Here's how the part is built. I have some questions about the finished solid (model axes, mm). Coordinates: 2 decimals unless noted, no trailing zeros. Loops run counter-clockwise (first coordinate to the right, second up) from the corner with the lowest first, then second, coordinate; pieces in that order, holes last. Notation, with made-up numbers: (52.5, -19) -> (109.5, -19) arc R6 ccw to (109.5, -12) -> close; hole circle Ø3 at (-16.75, -18). An arc over 180 degrees is marked (long way). Answer as a JSON object with one key per item and string values. Group by question number.
1) I want a section at B-B (x = 70). Write out the boundary of the cut face in (y, z), then the cut area to 3 significant figures.
2) I want a section at A-A (z = -120.5). Write out the boundary of the cut face in (x, y), then the cut area to 3 significant figures.
3) I want a section at C-C (y = -0.95). Count the separate pieces of the cut face and the enclosed holes in it, then the cut area to 3 significant figures.
4) I need wall thicknesses on probe 1 along X at (y, z) = (-0.5, -60); probe 2 along X at (y, z) = (-1.2, -145); probe 3 along Z at (x, y) = (181, -1.1). Which ranges of each line are inside material? Lowest first, please. Write a range as [from, to].
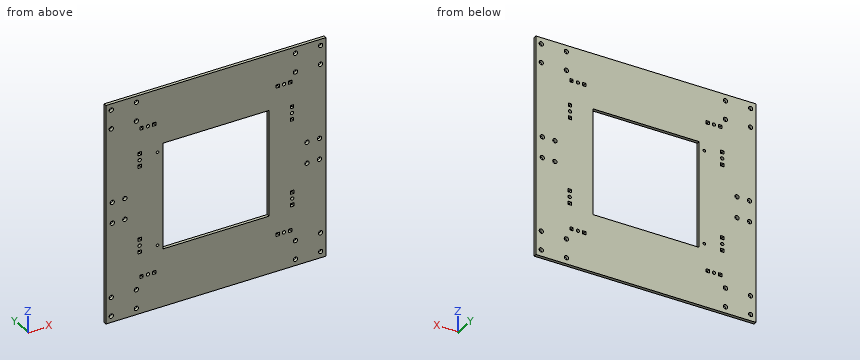
```python
from build123d import *

# Parameters (mm, degrees)
SKETCH2_W           = 210
SKETCH2_H           = 210
SKETCH2_R           = 2.05
SKETCH2_R_2         = 1.575
SKETCH2_R_3         = 1.25
SKETCH2_W_2         = 101.6
SKETCH2_H_2         = 101.6
SKETCH2_W_3         = 3.15
SKETCH2_H_3         = 3.15
BOSS_EXTRUDE2_DEPTH = 3


with BuildPart() as part:
    # Sketch2 → Boss-Extrude2 (new body)
    with BuildSketch(Plane(origin=(0, 0, 0), x_dir=(1, 0, 0), z_dir=(0, 1, 0))):
        with Locations((105, 105)):
            Rectangle(SKETCH2_W, SKETCH2_H)
        with Locations(Location((5, 24, 0), (0, 0, 270))):
            Circle(SKETCH2_R, mode=Mode.SUBTRACT)
        with Locations(Location((29, 24, 0), (0, 0, 270))):
            Circle(SKETCH2_R, mode=Mode.SUBTRACT)
        with Locations(Location((40, 32.3, 0), (0, 0, 270))):
            Circle(SKETCH2_R_2, mode=Mode.SUBTRACT)
        with Locations(Location((205, 6, 0), (0, 0, 270))):
            Circle(SKETCH2_R, mode=Mode.SUBTRACT)
        with Locations(Location((181, 6, 0), (0, 0, 270))):
            Circle(SKETCH2_R, mode=Mode.SUBTRACT)
        with Locations(Location((170, 32.3, 0), (0, 0, 270))):
            Circle(SKETCH2_R_2, mode=Mode.SUBTRACT)
        with Locations(Location((29, 6, 0), (0, 0, 270))):
            Circle(SKETCH2_R, mode=Mode.SUBTRACT)
        with Locations(Location((5, 6, 0), (0, 0, 270))):
            Circle(SKETCH2_R, mode=Mode.SUBTRACT)
        with Locations(Location((181, 24, 0), (0, 0, 270))):
            Circle(SKETCH2_R, mode=Mode.SUBTRACT)
        with Locations(Location((205, 24, 0), (0, 0, 270))):
            Circle(SKETCH2_R, mode=Mode.SUBTRACT)
        with Locations(Location((205, 186, 0), (0, 0, 270))):
            Circle(SKETCH2_R, mode=Mode.SUBTRACT)
        with Locations(Location((181, 186, 0), (0, 0, 270))):
            Circle(SKETCH2_R, mode=Mode.SUBTRACT)
        with Locations(Location((40, 174.76, 0), (0, 0, 270))):
            Circle(SKETCH2_R_2, mode=Mode.SUBTRACT)
        with Locations(Location((181, 204, 0), (0, 0, 270))):
            Circle(SKETCH2_R, mode=Mode.SUBTRACT)
        with Locations(Location((205, 204, 0), (0, 0, 270))):
            Circle(SKETCH2_R, mode=Mode.SUBTRACT)
        with Locations(Location((5, 204, 0), (0, 0, 270))):
            Circle(SKETCH2_R, mode=Mode.SUBTRACT)
        with Locations(Location((29, 204, 0), (0, 0, 270))):
            Circle(SKETCH2_R, mode=Mode.SUBTRACT)
        with Locations(Location((170, 174.76, 0), (0, 0, 270))):
            Circle(SKETCH2_R_2, mode=Mode.SUBTRACT)
        with Locations(Location((29, 186, 0), (0, 0, 270))):
            Circle(SKETCH2_R, mode=Mode.SUBTRACT)
        with Locations(Location((5, 186, 0), (0, 0, 270))):
            Circle(SKETCH2_R, mode=Mode.SUBTRACT)
        with Locations(Location((177.6, 62.41, 0), (0, 0, 270))):
            Circle(SKETCH2_R_2, mode=Mode.SUBTRACT)
        with Locations(Location((177.88, 144.65, 0), (0, 0, 270))):
            Circle(SKETCH2_R_2, mode=Mode.SUBTRACT)
        with Locations(Location((32.12, 144.65, 0), (0, 0, 270))):
            Circle(SKETCH2_R_2, mode=Mode.SUBTRACT)
        with Locations(Location((32.12, 62.41, 0), (0, 0, 270))):
            Circle(SKETCH2_R_2, mode=Mode.SUBTRACT)
        with Locations(Location((49.2, 149.719, 0), (0, 0, 270))):
            Circle(SKETCH2_R_3, mode=Mode.SUBTRACT)
        with Locations(Location((49.2, 60.281, 0), (0, 0, 270))):
            Circle(SKETCH2_R_3, mode=Mode.SUBTRACT)
        with Locations(Location((18.000065795, 95, 0), (0, 0, 270))):
            Circle(SKETCH2_R, mode=Mode.SUBTRACT)
        with Locations(Location((18, 115, 0), (0, 0, 270))):
            Circle(SKETCH2_R, mode=Mode.SUBTRACT)
        with Locations(Location((6, 115.000053284, 0), (0, 0, 270))):
            Circle(SKETCH2_R, mode=Mode.SUBTRACT)
        with Locations(Location((6, 95, 0), (0, 0, 270))):
            Circle(SKETCH2_R, mode=Mode.SUBTRACT)
        with Locations(Location((204, 95, 0), (0, 0, 270))):
            Circle(SKETCH2_R, mode=Mode.SUBTRACT)
        with Locations(Location((204, 115.000053284, 0), (0, 0, 270))):
            Circle(SKETCH2_R, mode=Mode.SUBTRACT)
        with Locations(Location((191.999934205, 95, 0), (0, 0, 270))):
            Circle(SKETCH2_R, mode=Mode.SUBTRACT)
        with Locations(Location((192, 115, 0), (0, 0, 270))):
            Circle(SKETCH2_R, mode=Mode.SUBTRACT)
        with Locations((105, 103.919)):
            Rectangle(SKETCH2_W_2, SKETCH2_H_2, mode=Mode.SUBTRACT)
        with Locations((32.12, 150.725)):
            Rectangle(SKETCH2_W_3, SKETCH2_H_3, mode=Mode.SUBTRACT)
        with Locations((32.12, 138.575)):
            Rectangle(SKETCH2_W_3, SKETCH2_H_3, mode=Mode.SUBTRACT)
        with Locations((32.12, 68.485)):
            Rectangle(SKETCH2_W_3, SKETCH2_H_3, mode=Mode.SUBTRACT)
        with Locations((32.12, 56.335)):
            Rectangle(SKETCH2_W_3, SKETCH2_H_3, mode=Mode.SUBTRACT)
        with Locations((177.6, 68.485)):
            Rectangle(SKETCH2_W_3, SKETCH2_H_3, mode=Mode.SUBTRACT)
        with Locations((177.6, 56.335)):
            Rectangle(SKETCH2_W_3, SKETCH2_H_3, mode=Mode.SUBTRACT)
        with Locations((177.88, 138.575)):
            Rectangle(SKETCH2_W_3, SKETCH2_H_3, mode=Mode.SUBTRACT)
        with Locations((177.88, 150.725)):
            Rectangle(SKETCH2_W_3, SKETCH2_H_3, mode=Mode.SUBTRACT)
        with Locations((33.925, 32.3)):
            Rectangle(SKETCH2_W_3, SKETCH2_H_3, mode=Mode.SUBTRACT)
        with Locations((46.075, 32.3)):
            Rectangle(SKETCH2_W_3, SKETCH2_H_3, mode=Mode.SUBTRACT)
        with Locations((33.925, 174.76)):
            Rectangle(SKETCH2_W_3, SKETCH2_H_3, mode=Mode.SUBTRACT)
        with Locations((46.075, 174.76)):
            Rectangle(SKETCH2_W_3, SKETCH2_H_3, mode=Mode.SUBTRACT)
        with Locations((176.075, 32.3)):
            Rectangle(SKETCH2_W_3, SKETCH2_H_3, mode=Mode.SUBTRACT)
        with Locations((163.925, 32.3)):
            Rectangle(SKETCH2_W_3, SKETCH2_H_3, mode=Mode.SUBTRACT)
        with Locations((163.925, 174.76)):
            Rectangle(SKETCH2_W_3, SKETCH2_H_3, mode=Mode.SUBTRACT)
        with Locations((176.075, 174.76)):
            Rectangle(SKETCH2_W_3, SKETCH2_H_3, mode=Mode.SUBTRACT)
    extrude(amount=-BOSS_EXTRUDE2_DEPTH)


solid = part.part
```
Determined:
{
 "1": {"outline": "(-3, -210) -> (0, -210) -> (0, -154.72) -> (-3, -154.72) -> close; (-3, -53.12) -> (0, -53.12) -> (0, 0) -> (-3, 0) -> close", "area": "325 mm^2"},
 "2": {"outline": "(0, -3) -> (54.2, -3) -> (54.2, 0) -> (0, 0) -> close; (155.8, -3) -> (210, -3) -> (210, 0) -> (155.8, 0) -> close", "area": "325 mm^2"},
 "3": {"separate pieces": "1", "enclosed holes": "51", "area": "33,200 mm^2"},
 "4": {"probe 1": "[0, 47.98], [50.42, 54.2], [155.8, 210]", "probe 2": "[0, 30.58], [33.66, 54.2], [155.8, 176.34], [179.42, 210]", "probe 3": "[-210, -206.05], [-201.95, -188.05], [-183.95, -26.05], [-21.95, -8.05], [-3.95, 0]"}
}
